For this review, use the dimensioned drawing (mm, ordinates from the lowest corner) and the shaded views. A direction names the side the tool comes from. Round coordinates to 2 decimals unless told otherwise and drop trailing zeros. Write each loop counter-clockwise with the first axis right and the second up, starting at its lowest first coordinate (ties: lowest second). Pieces come first, ordered by that corner, then holes. Notation, with made-up numbers: M 72,2.25 L 103,2.25 A34 ccw 103,39.25 Z; hole C -19.75,73 d10. An arc over 180 degrees is marked long. Answer in a Markdown table with one row per item.
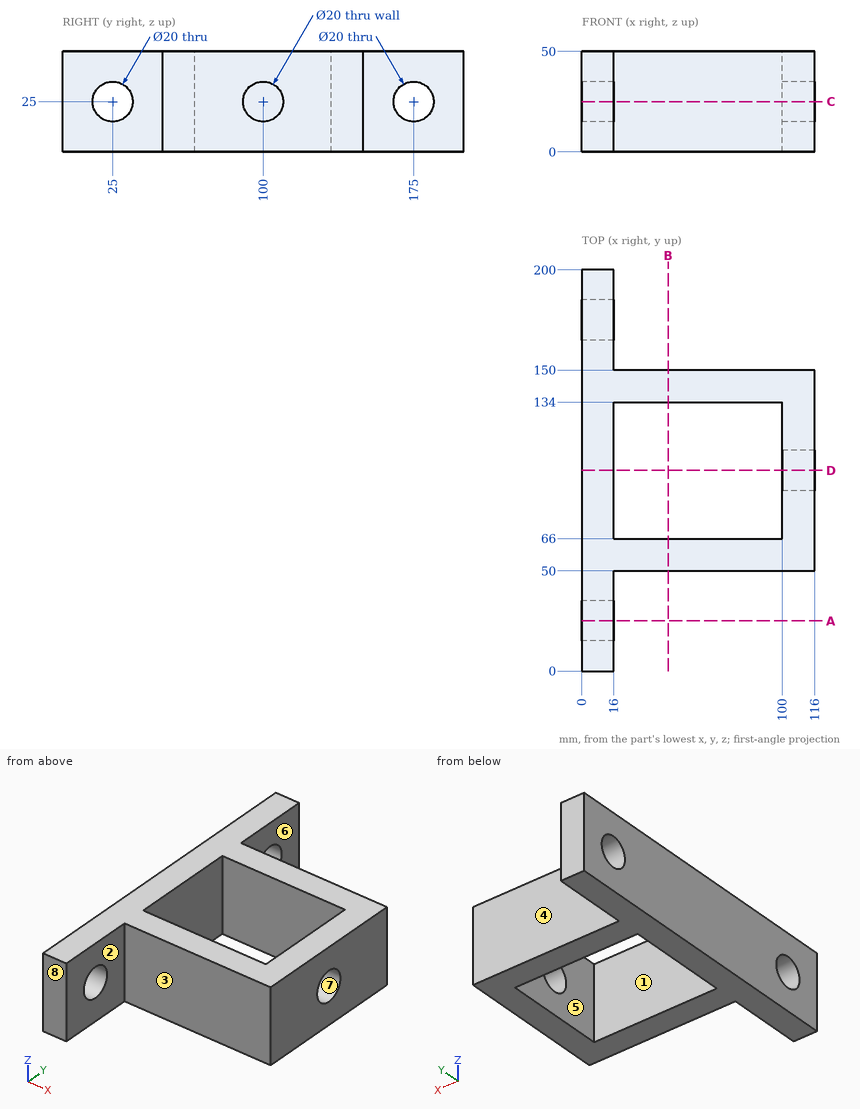
Q1. Take a section at D-D (y = 100). State the section outline as (x, z) points, then the cut area to 3 significant figures.
Found:
| item | result |
|---|---|
| outline | M 0,0 L 16,0 L 16,50 L 0,50 Z; M 100,0 L 116,0 L 116,15 L 100,15 Z; M 100,35 L 116,35 L 116,50 L 100,50 Z |
| area | 1,280 mm² |
Q2. Take a section at B-B (x = 43). State the section outline as (y, z) points, then the cut area to 3 significant figures.
Found:
| item | result |
|---|---|
| outline | M 50,0 L 66,0 L 66,50 L 50,50 Z; M 134,0 L 150,0 L 150,50 L 134,50 Z |
| area | 1,600 mm² |
Q3. Mouldability with a two-part tool opening along Y and no side actions: class the marked faces 1, 2, 3 and 4 as +Y half, -Y half, draft (parallel to the pull), parting line (faces both ways), or undercut.
Found:
| item | result |
|---|---|
| face 1 | undercut |
| face 2 | draft |
| face 3 | -Y half |
| face 4 | +Y half |
Q4. For probe 1 along Z at (x, y) = (104.5, 100); probe 2 along Y at (x, z) = (58, 6.5); probe 3 along X at (y, z) = (94, 5), list the stretches that pass through material, from the lowest coordinate up.
Found:
| item | result |
|---|---|
| probe 1 | 0 to 15, 35 to 50 |
| probe 2 | 50 to 66, 134 to 150 |
| probe 3 | 0 to 16, 100 to 116 |
Q5. Insertion check: P1, Ø25, axis at x = 71.5, z = 29.5, coming from the +Y side; P2, Ø16, axis at y = 100, z = 25, coming from the +X side; P3, Ø15, axis at y = 91.5, z = 28, coming from the +X side; P4, Ø5, axis at x = 96.5, z = 37, coming from the -Y side. Each pin has a flat end and moves straight along its axis. Give the tip position at first contact, or say it passes through.
Found:
| item | result |
|---|---|
| P1 | y = 150 |
| P2 | x = 16 |
| P3 | x = 116 |
| P4 | y = 50 |
Q6. Machinability: for the marked faces 5, 6, 7 and 8, which of the approach directions +Z, -Z, +X, -X, +Y, -Y give a long, thin tool a straight path to every point of the face, cutting with its end or side? Answer none if there is none.
Found:
| item | result |
|---|---|
| face 5 | +Z, -Z |
| face 6 | +Z, -Z, +X, +Y |
| face 7 | +X |
| face 8 | +Z, -Z, +X, -X, -Y |
Q7. Take a section at C-C (z = 25). State the section outline as (x, y) points, then the cut area to 3 significant figures.
Found:
| item | result |
|---|---|
| outline | M 0,0 L 16,0 L 16,15 L 0,15 Z; M 0,35 L 16,35 L 16,50 L 116,50 L 116,90 L 100,90 L 100,66 L 16,66 L 16,134 L 100,134 L 100,110 L 116,110 L 116,150 L 16,150 L 16,165 L 0,165 Z; M 0,185 L 16,185 L 16,200 L 0,200 Z |
| area | 6,530 mm² |
Q8. Take a section at A-A (y = 25). State the section outline as (x, z) points, then the cut area to 3 significant figures.
Found:
| item | result |
|---|---|
| outline | M 0,0 L 16,0 L 16,15 L 0,15 Z; M 0,35 L 16,35 L 16,50 L 0,50 Z |
| area | 480 mm² |
